The drawing under review shows one solid part. Ordinate dimensions are in mm from its lowest x, y, z. Round coordinates to 2 decimals unless told otherwise and drop trailing zeros. Write each loop counter-clockwise with the first axis right and the second up, starting at its lowest first coordinate (ties: lowest second). Pieces come first, ordered by that corner, then holes. Notation, with made-up numbers: (12.5, 86.5) -> (31.5, 86.5) arc R16 cw to (31.5, 110.5) -> close; hole circle Ø8 at (17.25, 38). An arc over 180 degrees is marked (long way). Answer in a Markdown table with one row per item.
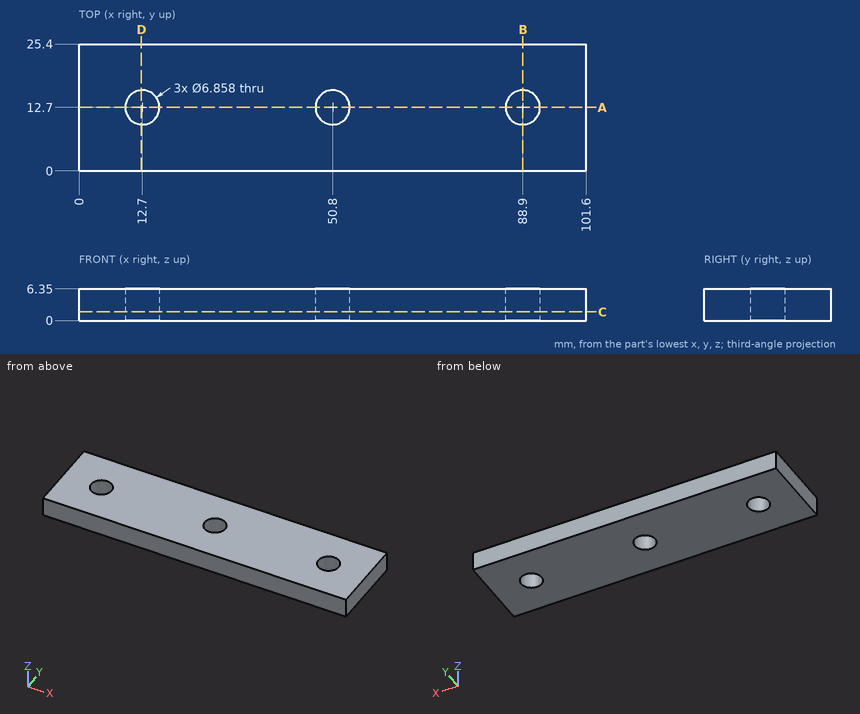
1) Consider section C-C on z = 1.75. State the section outline as (x, y) points, then the cut area to 3 significant figures.
Solved:
| item | result |
|---|---|
| outline | (0, 0) -> (101.6, 0) -> (101.6, 25.4) -> (0, 25.4) -> close; hole circle Ø6.86 at (12.7, 12.7); hole circle Ø6.86 at (50.8, 12.7); hole circle Ø6.86 at (88.9, 12.7) |
| area | 2,470 mm² |
2) Consider section A-A on y = 12.7. State the section outline as (x, z) points, then the cut area to 3 significant figures.
Solved:
| item | result |
|---|---|
| outline | (0, 0) -> (9.27, 0) -> (9.27, 6.35) -> (0, 6.35) -> close; (16.13, 0) -> (47.37, 0) -> (47.37, 6.35) -> (16.13, 6.35) -> close; (54.23, 0) -> (85.47, 0) -> (85.47, 6.35) -> (54.23, 6.35) -> close; (92.33, 0) -> (101.6, 0) -> (101.6, 6.35) -> (92.33, 6.35) -> close |
| area | 515 mm² |
3) For line 1 (X direction, y = 11, z = 4); line 2 (Y direction, x = 12.7, z = 4.25); line 3 (X direction, y = 13.5, z = 2.5), list the stretches that pass through material, from the lowest coordinate up. Write a range as [from, to].
Solved:
| item | result |
|---|---|
| line 1 | [0, 9.72], [15.68, 47.82], [53.78, 85.92], [91.88, 101.6] |
| line 2 | [0, 9.27], [16.13, 25.4] |
| line 3 | [0, 9.37], [16.03, 47.47], [54.13, 85.57], [92.23, 101.6] |
4) Consider section B-B on x = 88.9. State the section outline as (y, z) points, then the cut area to 3 significant figures.
Solved:
| item | result |
|---|---|
| outline | (0, 0) -> (9.27, 0) -> (9.27, 6.35) -> (0, 6.35) -> close; (16.13, 0) -> (25.4, 0) -> (25.4, 6.35) -> (16.13, 6.35) -> close |
| area | 118 mm² |
5) Clearance check with a flat-ended pin moving along its axis: pin 1 Ø5.5 at (x, y) = (12.7, 12.7) entering from +Z. State where the tip first meets the part, or that it passes through.
Solved:
| item | result |
|---|---|
| pin 1 | through |
6) Consider section D-D on x = 12.5. State the section outline as (y, z) points.
Solved:
| item | result |
|---|---|
| outline | (0, 0) -> (9.28, 0) -> (9.28, 6.35) -> (0, 6.35) -> close; (16.12, 0) -> (25.4, 0) -> (25.4, 6.35) -> (16.12, 6.35) -> close |
